Work out the finished part from the listing and answer in its coordinate system (mm). A direction names the side the tool comes from. Coordinates: 2 decimals unless noted, no trailing zeros. Write each loop counter-clockwise with the first axis right and the second up, starting at its lowest first coordinate (ties: lowest second). Pieces come first, ordered by that corner, then holes. Notation, with made-up numbers: M 40,65 L 52,65 A20 ccw 52,92 Z; hole C -33,48.25 d4. An arc over 180 degrees is marked long. Answer as CSV lines item,"result". Start each with the question number.
(1) A cutting plane is placed at D-D on x = 11.25. Give the vertices of the cut face in (y, z), then the cut area to 3 significant figures.
(2) A cutting plane is placed at B-B on z = -9.25. Give the vertices of the cut face in (x, y), then the cut area to 3 significant figures.
(3) For faces 1 (the flat face through (0, -16.6, 4)), 2 (the flat face through (-9.76, -4.2, -6.14)), 3 (the flat face through (0, -15.201, -7)), 4 (the flat face through (7.65, 0, 4)), 5 (the flat face through (11, -4, 0)), determine the directions among +Z, -Z, +X, -X, +Y, -Y from which every point of the face is accessible in a straight line to the end or side of a thin tool.
(4) Flat-ended cylindrical pins translate along their axes: P1, Ø2.5, axis at x = -11.25, z = 3.58, coming from the +Y side; P2, Ø1.1, axis at x = 1, y = -21.5, coming from the +Z side; P3, Ø3, axis at y = -11.5, z = -2, coming from the -X side; P4, Ø2, axis at y = -4.5, z = -8, coming from the -X side. Find the tip coordinate at first contact, or state that the pin passes through.
(5) A cutting plane is placed at C-C on y = 14.1. Give the vertices of the cut face in (x, z).
(6) Find the intervals of material crossed by L1, parallel to X at y = -1, z = 3.75; L2, parallel to X at y = 11, z = 3.5; L3, parallel to Y at x = -2, z = 4.5, in increasing order. Write a range as [from, to].
(7) The mould has two halves that part along Z. Classify faces 6 (the flat face through (0, 0, 2)), 7 (the flat face through (-11, -4, 0)), 8 (the cylindrical face through (0.877, 12.414, 4.042)): released by +Z, released by -Z, zero draft, split by the parting line, or undercut.
(8) A cutting plane is placed at A-A on x = 0. Count the separate pieces of the cut face and the enclosed holes in it, then the cut area to 3 significant figures.
from build123d import *

# Parameters (mm, degrees)
SKETCH_2_W               = 31.3
SKETCH_2_H               = 34.2
SKETCH_2_W_2             = 15.3
SKETCH_2_H_2             = 21.2
EXTRUDE_1_DEPTH          = 7
SKETCH_2_3_W             = 15.3
SKETCH_2_3_H             = 21.2
EXTRUDE_2_DEPTH          = 2
SKETCH_5_W               = 7.971023584
SKETCH_5_H               = 4.648657004
CUT_EXTRUDE_2_DEPTH      = 7
CUT_EXTRUDE_3_DEPTH      = 39.256535389
CUT_EXTRUDE_3_DEPTH_BACK = 39.256535389
SKETCH_6_R               = 1.9
EXTRUDE_3_DEPTH          = 34.2
SKETCH_8_R               = 1.9
CUT_EXTRUDE_4_DEPTH      = 6
SKETCH_9_W               = 7.971023584
SKETCH_9_H               = 8.623939395
CUT_EXTRUDE_5_DEPTH      = 28.63322883
EXTRUDE_START            = 8.8
SKETCH_10_R              = 1.9
EXTRUDE_4_DEPTH          = 8.8
CUT_EXTRUDE_6_DEPTH      = 36.616478053
CUT_EXTRUDE_6_DEPTH_BACK = 8
SKETCH_11_R              = 1.9
CUT_EXTRUDE_7_DEPTH      = 48.423834368
CUT_EXTRUDE_7_DEPTH_BACK = 48.423834368
SKETCH_12_R              = 1.9


with BuildPart() as part:
    # 草图2 → 凸台-拉伸1 (new body)
    with BuildSketch(Plane.XY):
        with Locations((0, 0.5)):
            Rectangle(SKETCH_2_W, SKETCH_2_H)
        Rectangle(SKETCH_2_W_2, SKETCH_2_H_2, mode=Mode.SUBTRACT)
    extrude(amount=EXTRUDE_1_DEPTH)

    # 草图2<3> → 凸台-拉伸2 (add)
    with BuildSketch(Plane.XY):
        Rectangle(SKETCH_2_3_W, SKETCH_2_3_H)
    extrude(amount=EXTRUDE_2_DEPTH)

    # 草图5 → 切除-拉伸2 (cut)
    with BuildSketch(Plane(origin=(0, -10.6, 0), x_dir=(1, 0, 0), z_dir=(0, 1, 0))):
        with Locations((0, -3.548249301)):
            Rectangle(SKETCH_5_W, SKETCH_5_H)
    extrude(amount=-CUT_EXTRUDE_2_DEPTH, mode=Mode.SUBTRACT)

    # 草图6 → 切除-拉伸3 (cut, two sides: drawn at the far end of the back side and taken through both)
    with BuildSketch(Plane.XZ.offset(16.6).offset(-CUT_EXTRUDE_3_DEPTH_BACK)):
        with Locations((-11.25, 3.583357856)):
            Circle(SKETCH_6_R)
        with Locations(Location((11.25, 3.583357856, 0), (0, 0, 180))):
            Circle(SKETCH_6_R)
    extrude(amount=CUT_EXTRUDE_3_DEPTH + CUT_EXTRUDE_3_DEPTH_BACK, mode=Mode.SUBTRACT)

    # 草图7 → 凸台-拉伸3 (add)
    with BuildSketch(Plane.XZ.offset(16.6)):
        Polygon((7.118714005, 0), (-7.118714005, 0), (-12.476482967, -12.453817335), (12.476482967, -12.453817335), align=None)
    extrude(amount=-EXTRUDE_3_DEPTH)

    # 草图8 → 切除-拉伸4 (cut)
    with BuildSketch(Plane.XY.offset(7)):
        with Locations((0, 14.1)):
            Circle(SKETCH_8_R)
    extrude(amount=-CUT_EXTRUDE_4_DEPTH, mode=Mode.SUBTRACT)

    # 草图9 → 切除-拉伸5 (cut, through all)
    with BuildSketch(Plane.XY.offset(2)):
        with Locations((0, -10.888708642)):
            Rectangle(SKETCH_9_W, SKETCH_9_H)
    extrude(amount=-CUT_EXTRUDE_5_DEPTH, mode=Mode.SUBTRACT)

    # 草图10 → 凸台-拉伸4 (add)
    with BuildSketch(Plane.XZ.offset(16.6).offset(EXTRUDE_START)):
        Polygon((-15.65, 7), (-15.65, 0), (-7.118714005, 0), (-12.476482967, -12.453817335), (12.476482967, -12.453817335), (7.118714005, 0), (15.65, 0), (15.65, 7), align=None)
        with Locations((-11.25, 3.583357856)):
            Circle(SKETCH_10_R, mode=Mode.SUBTRACT)
        with Locations((11.25, 3.583357856)):
            Circle(SKETCH_10_R, mode=Mode.SUBTRACT)
    extrude(amount=-EXTRUDE_4_DEPTH)

    # 草图11 → 切除-拉伸6 (cut, two sides: drawn at the far end of the back side and taken through both)
    with BuildSketch(Plane.XY.offset(7).offset(-CUT_EXTRUDE_6_DEPTH_BACK)):
        with Locations(Location((0, -21.063101394, 0), (0, 0, 180))):
            Circle(SKETCH_11_R)
    extrude(amount=CUT_EXTRUDE_6_DEPTH + CUT_EXTRUDE_6_DEPTH_BACK, mode=Mode.SUBTRACT)

    # 草图12 → 切除-拉伸7 (cut, two sides: drawn at the far end of the back side and taken through both)
    with BuildSketch(Plane.XZ.offset(25.4).offset(-CUT_EXTRUDE_7_DEPTH_BACK)):
        with Locations((0, -4.727248667)):
            Circle(SKETCH_12_R)
    extrude(amount=CUT_EXTRUDE_7_DEPTH + CUT_EXTRUDE_7_DEPTH_BACK, mode=Mode.SUBTRACT)


solid = part.part
Here are the results:
1,outline,"M -25.4,-12.45 L 17.6,-12.45 L 17.6,-9.6 L -25.4,-9.6 Z; M -25.4,0 L 17.6,0 L 17.6,1.68 L -25.4,1.68 Z; M -25.4,5.48 L 17.6,5.48 L 17.6,7 L -25.4,7 Z"
1,area,"260 mm^2"
2,outline,"M -11.1,-25.4 L 11.1,-25.4 L 11.1,17.6 L -11.1,17.6 Z; hole M -3.99,-15.2 L 3.99,-15.2 L 3.99,-6.58 L -3.99,-6.58 Z"
2,area,"886 mm^2"
3,face 1,"none"
3,face 2,"-X, +Y, -Y"
3,face 3,"-Z"
3,face 4,"+Z"
3,face 5,"+X, +Y, -Y"
4,P1,"passes through"
4,P2,"stops at z = -1"
4,P3,"stops at x = -8.62"
4,P4,"stops at x = -10.99"
5,outline,"M -15.65,0 L -7.12,0 L -12.48,-12.45 L 12.48,-12.45 L 7.12,0 L 15.65,0 L 15.65,7 L 1.9,7 L 1.9,1 L -1.9,1 L -1.9,7 L -15.65,7 Z; hole C -11.25,3.58 d3.8; hole C 0,-4.73 d3.8; hole C 11.25,3.58 d3.8"
6,L1,"x = [-15.65, -13.14], [-9.36, -7.65], [7.65, 9.36], [13.14, 15.65]"
6,L2,"x = [-15.65, -13.15], [-9.35, 9.35], [13.15, 15.65]"
6,L3,"y = [-25.4, -16.6], [10.6, 17.6]"
7,face 6,"released by +Z"
7,face 7,"undercut"
7,face 8,"zero draft"
8,separate pieces,"4"
8,enclosed holes,"0"
8,area,"398 mm^2"
